Source: CAD feature listing. Evaluate the final solid. Frame: model axes, mm. Face numbers are marked on the shaded views. Give positions to 0.01 mm unless a question says otherwise; leave off trailing zeros. Order: outer loops, then holes, each group sorted by start corner. A loop starts at its lowest first (then second) coordinate and runs counter-clockwise, first axis right, second up. Notation, with made-up numbers: M 70,57 L 85,57 A20 cw 85,65 Z; hole C -12,-27.75 d7. An arc over 180 degrees is marked long. Answer as a JSON object with one key per item and string values. Group by question number.
1. Section query C-C (z = 41). Output: boundary loops of the cut face in (x, y).
2. Section query A-A (y = 0). Output: boundary loops of the cut face in (x, z), plus the area to 3 significant figures.
3. Pull-direction query (Y, two-part tool) for the marked faces 1, 2 and 3; classes: +Y half, -Y half, draft (parallel to the pull), parting line (faces both ways), or undercut.
4. Pin query (flat end, axial travel): P1, Ø19.5, axis at x = 7, y = -0.5, coming from the +Z side; P2, Ø10, axis at x = 5, y = -18, coming from the +Z side; P3, Ø3, axis at x = 1.5, z = 75.5, coming from the -Y side; P4, Ø12, axis at x = 25.5, z = 80, coming from the -Y side (3 decimals). Return the tip coordinate at first contact, or that it passes through.
5. Material intervals for L1, parallel to Z at x = 14, y = -8.5; L2, parallel to Y at x = -29.5, z = 5.25; L3, parallel to X at y = -4, z = 30, sorted ascending. Write a range as [from, to].
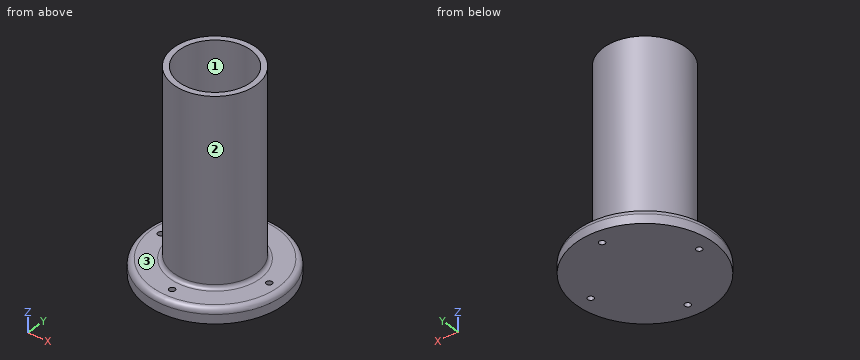
from build123d import *

# Parameters (mm, degrees)
SZKIC1_R                    = 37.5
SZKIC1_R_2                  = 1.6
DODANIE_WYCI_GNI_CIE1_DEPTH = 8
ZAOKR_GLENIE1_R             = 3
SZKIC2_R                    = 22.5
SZKIC2_R_2                  = 19.5
DODANIE_WYCI_GNI_CIE2_DEPTH = 100
ZAOKR_GLENIE2_R             = 2


with BuildPart() as part:
    # Szkic1 → Dodanie-wyciągnięcie1 (new body)
    with BuildSketch(Plane.XY):
        Circle(SZKIC1_R)
        with Locations((0, 29.5)):
            Circle(SZKIC1_R_2, mode=Mode.SUBTRACT)
        with Locations((29.5, 0)):
            Circle(SZKIC1_R_2, mode=Mode.SUBTRACT)
        with Locations((0, -29.5)):
            Circle(SZKIC1_R_2, mode=Mode.SUBTRACT)
        with Locations((-29.5, 0)):
            Circle(SZKIC1_R_2, mode=Mode.SUBTRACT)
    extrude(amount=DODANIE_WYCI_GNI_CIE1_DEPTH)

    # Zaokrąglenie1
    zaokr_glenie1_edges = [part.edges().sort_by_distance(p)[0] for p in [
        (-37.5, 0, 8),
    ]]
    fillet(zaokr_glenie1_edges, radius=ZAOKR_GLENIE1_R)

    # Szkic2 → Dodanie-wyciągnięcie2 (add)
    with BuildSketch(Plane.XY.offset(8)):
        Circle(SZKIC2_R)
        Circle(SZKIC2_R_2, mode=Mode.SUBTRACT)
    extrude(amount=DODANIE_WYCI_GNI_CIE2_DEPTH)

    # Zaokrąglenie2
    zaokr_glenie2_edges = [part.edges().sort_by_distance(p)[0] for p in [
        (-22.5, 0, 8),
    ]]
    fillet(zaokr_glenie2_edges, radius=ZAOKR_GLENIE2_R)


solid = part.part
Answer sheet:
{
 "1": {"outline": "C 0,0 d45; hole C 0,0 d39"},
 "2": {"outline": "M -37.5,0 L -31.1,0 L -31.1,8 L -34.5,8 A3 ccw -37.5,5 Z; M -27.9,0 L 27.9,0 L 27.9,8 L 24.5,8 A2 cw 22.5,10 L 22.5,108 L 19.5,108 L 19.5,8 L -19.5,8 L -19.5,108 L -22.5,108 L -22.5,10 A2 cw -24.5,8 L -27.9,8 Z; M 31.1,0 L 37.5,0 L 37.5,5 A3 ccw 34.5,8 L 31.1,8 Z", "area": "1,150 mm^2"},
 "3": {"face 1": "undercut", "face 2": "parting line", "face 3": "draft"},
 "4": {"P1": "z = 8", "P2": "z = 108", "P3": "y = -22.5", "P4": "y = -11.225"},
 "5": {"L1": "[0, 8]", "L2": "[-23.13, -1.6], [1.6, 23.13]", "L3": "[-22.14, -19.09], [19.09, 22.14]"}
}
